Could you check a few things on this model? Use its own coordinates, in mm. A direction names the side the tool comes from. Give positions to 0.01 mm unless a question says otherwise; leave off trailing zeros. Order: outer loops, then holes, each group sorted by start corner. A loop starts at its lowest first (then second) coordinate and runs counter-clockwise, first axis right, second up.
from build123d import *

# Parameters (mm, degrees)
ESQUISSE1_R          = 1
BASE_EXTRUSION_DEPTH = 1.5


with BuildPart() as part:
    # Esquisse1 → Base-Extrusion (new body)
    with BuildSketch(Plane.XY):
        with BuildLine():
            Line((5.564558924, -20.767216626), (4.837312367, -18.053095527))
            ThreePointArc((4.837312367, -18.053095527), (4.924160237, -17.31759845), (5.493181049, -16.84355856))
            ThreePointArc((5.493181049, -16.84355856), (8.858336511, -15.343088908), (11.840359078, -13.179013616))
            ThreePointArc((11.840359078, -13.179013616), (12.535400072, -12.923247082), (13.215783159, -13.215783159))
            Line((13.215783159, -13.215783159), (14.566399692, -14.566399692))
            ThreePointArc((14.566399692, -14.566399692), (0, 20.6), (-14.566399692, -14.566399692))
            Line((-14.566399692, -14.566399692), (-13.215783159, -13.215783159))
            ThreePointArc((-13.215783159, -13.215783159), (-12.535400072, -12.923247082), (-11.840359078, -13.179013616))
            ThreePointArc((-11.840359078, -13.179013616), (-8.858336511, -15.343088908), (-5.493181049, -16.84355856))
            ThreePointArc((-5.493181049, -16.84355856), (-4.924160237, -17.31759845), (-4.837312367, -18.053095527))
            Line((-4.837312367, -18.053095527), (-5.564558924, -20.767216626))
            ThreePointArc((-5.564558924, -20.767216626), (-6.047721334, -21.384148392), (-6.827324966, -21.463324744))
            ThreePointArc((-6.827324966, -21.463324744), (0, 23.5), (6.827324966, -21.463324744))
            ThreePointArc((6.827324966, -21.463324744), (6.047721334, -21.384148392), (5.564558924, -20.767216626))
        make_face()
        with Locations((-9.883667669, -16.988277884)):
            Circle(ESQUISSE1_R, mode=Mode.SUBTRACT)
        with Locations(Location((9.883667669, -16.988277884, 0), (0, 0, 180))):
            Circle(ESQUISSE1_R, mode=Mode.SUBTRACT)
    extrude(amount=BASE_EXTRUSION_DEPTH)


solid = part.part
Item 1: Imagine slicing it at B-B on z = 0.9. List the corners of the cut face in (x, y) for me, then the cut area to 3 significant figures.
Findings:
outline: (-14.57, -14.57) arc R20.6 cw (long way) to (14.57, -14.57) - (13.22, -13.22) arc R1 ccw to (11.84, -13.18) arc R17.72 cw to (5.49, -16.84) arc R1 ccw to (4.84, -18.05) - (5.56, -20.77) arc R1 ccw to (6.83, -21.46) arc R23 ccw (long way) to (-6.83, -21.46) arc R1 ccw to (-5.56, -20.77) - (-4.84, -18.05) arc R1 ccw to (-5.49, -16.84) arc R17.72 cw to (-11.84, -13.18) arc R1 ccw to (-13.22, -13.22) - close; hole circle Ø2 at (-9.88, -16.99); hole circle Ø2 at (9.88, -16.99)
area: 358 mm2
Item 2: Imagine slicing it at A-A on y = 2.5. List the corners of the cut face in (x, z) for me, then the cut area to 3 significant figures.
Findings:
outline: (-22.91, 0) - (-20.45, 0) - (-20.45, 1.5) - (-22.91, 1.5) - close; (20.45, 0) - (22.91, 0) - (22.91, 1.5) - (20.45, 1.5) - close
area: 7.40 mm2
Item 3: We'd pull the mould along Y, two halves only. Please class faces 4 (the flat face through (-14, -14, 1)), 5 (the flat face through (5.2, -19.4, 0.7)), 6 (the flat face through (9, -16, 1.5)), 7 (the cylindrical face through (-4.93, -17.31, 0.74)): +Y half, -Y half, draft (parallel to the pull), parting line (faces both ways), or undercut.
Findings:
face 4: undercut
face 5: -Y half
face 6: draft
face 7: undercut
Item 4: Imagine slicing it at D-D on x = 0. List the corners of the cut face in (y, z) for me.
Findings:
outline: (20.6, 0) - (23.5, 0) - (23.5, 1.5) - (20.6, 1.5) - close
Item 5: Please list where these lines run through material, in increasing order: line 1 along X through (y, z) = (0, 0.2); line 2 along Y through (x, z) = (10, 0.95); line 3 along X through (y, z) = (7.5, 0.5).
Findings:
line 1: x = -22.99 to -20.6, 20.6 to 22.99
line 2: y = -20.21 to -17.98, -16 to -14.62, 18.01 to 21.21
line 3: x = -21.91 to -19.19, 19.19 to 21.91
Item 6: Imagine slicing it at C-C on x = -16.5. List the corners of the cut face in (y, z) for me, then the cut area to 3 significant figures.
Findings:
outline: (-15.52, 0) - (-12.33, 0) - (-12.33, 1.5) - (-15.52, 1.5) - close; (12.33, 0) - (16.52, 0) - (16.52, 1.5) - (12.33, 1.5) - close
area: 11.1 mm2
Item 7: For faces 1 (the flat face through (-5.2, -19.4, 0.7)), 2 (the flat face through (9, -16, 0)), 3 (the cylindrical face through (-12.546, -12.924, 0.74)), which set-ups out of +Z, -Z, +X, -X, +Y, -Y let a thin tool reach every point of the face, with its end or its side?
Findings:
face 1: +Z, -Z, -Y
face 2: -Z, +X, -X, +Y, -Y
face 3: +Z, -Z
Item 8: For pin 1 (3 mm diameter, centred on x = -9.88, y = -16.99, fed in from +Z), with a flat end and sliding along its axis, tell me the tip position at first contact or that it passes through.
Findings:
pin 1: stops at z = 1.5
